from build123d import *

# Parameters (mm, degrees)
BOSS_EXTRUDE1_DEPTH = 10
SKETCH2_R           = 2.5
CUT_EXTRUDE1_DEPTH  = 10
SKETCH4_R           = 1.7
CUT_EXTRUDE4_DEPTH  = 20
CHAMFER1_SIZE       = 2.5
CHAMFER2_SIZE       = 1


with BuildPart() as part:
    # Sketch1 → Boss-Extrude1 (new body)
    with BuildSketch(Plane(origin=(0, 0, 0), x_dir=(1, 0, 0), z_dir=(0, 1, 0))):
        Polygon((-5, 5), (-5, 3), (-30, 3), (-30, -3), (-5, -3), (-5, -5), (5, -5), (5, 5), align=None)
    extrude(amount=BOSS_EXTRUDE1_DEPTH)

    # Sketch2 → Cut-Extrude1 (cut)
    with BuildSketch(Plane(origin=(0, 10, 0), x_dir=(1, 0, 0), z_dir=(0, 1, 0))):
        with Locations(Location((0, 0, 0), (0, 0, 270))):
            Circle(SKETCH2_R)
    extrude(amount=-CUT_EXTRUDE1_DEPTH, mode=Mode.SUBTRACT)

    # Sketch4 → Cut-Extrude4 (cut)
    with BuildSketch(Plane.ZY.offset(30)):
        with Locations((0, 5)):
            Circle(SKETCH4_R)
    extrude(amount=-CUT_EXTRUDE4_DEPTH, mode=Mode.SUBTRACT)

    # Chamfer1
    # the kernel refuses this chamfer: 2.5 mm, written as the material it takes off along each edge
    with BuildSketch(Plane(origin=(5, -6.42920747, -5), x_dir=(-0.9996219169112968, 0, -0.027495876610586317), z_dir=(0, 1, 0)), Plane(origin=(5, -6.42920747, 5), x_dir=(0.027495876610586317, 0, -0.9996219169112968), z_dir=(0, 1, 0))) as chamfer1_piece_1:
        Polygon((CHAMFER1_SIZE * 0.999621916911, CHAMFER1_SIZE * 0.0274958766106), (-CHAMFER1_SIZE * 0.0274958766106, CHAMFER1_SIZE * 0.999621916911), (0, 0), align=None)
    extrude(amount=22.85841494, mode=Mode.SUBTRACT)
    with BuildSketch(Plane(origin=(-5, -6.42920747, 5), x_dir=(0.9996219169112968, 0, 0.027495876610586317), z_dir=(0, 1, 0))) as chamfer1_piece_2_section:
        Polygon((CHAMFER1_SIZE * 0.999621916911, CHAMFER1_SIZE * 0.0274958766106), (-CHAMFER1_SIZE * 0.0274958766106, CHAMFER1_SIZE * 0.999621916911), (0, 0), align=None)
    chamfer1_piece_2 = extrude(amount=22.85841494, mode=Mode.PRIVATE)
    chamfer1_piece_2 = split(chamfer1_piece_2, bisect_by=Plane(origin=(-4.135703969, 5, 3), z_dir=(0, 0, 1)), keep=Keep.TOP, mode=Mode.PRIVATE)
    add(chamfer1_piece_2, mode=Mode.SUBTRACT)
    with BuildSketch(Plane(origin=(-5, -6.42920747, -5), x_dir=(-0.027495876610588735, 0, 0.9996219169112968), z_dir=(0, 1, 0))) as chamfer1_piece_3_section:
        Polygon((CHAMFER1_SIZE * 0.999621916911, CHAMFER1_SIZE * 0.0274958766106), (-CHAMFER1_SIZE * 0.0274958766106, CHAMFER1_SIZE * 0.999621916911), (0, 0), align=None)
    chamfer1_piece_3 = extrude(amount=22.85841494, mode=Mode.PRIVATE)
    chamfer1_piece_3 = split(chamfer1_piece_3, bisect_by=Plane(origin=(-4.135703969, 5, -3), z_dir=(0, 0, -1)), keep=Keep.TOP, mode=Mode.PRIVATE)
    add(chamfer1_piece_3, mode=Mode.SUBTRACT)

    # Chamfer2
    chamfer2_edges = [part.edges().sort_by_distance(p)[0] for p in [
        (-17.25, 10, -3),
        (-17.25, 10, 3),
        (-17.25, 0, 3),
        (-17.25, 0, -3),
    ]]
    chamfer(chamfer2_edges, length=CHAMFER2_SIZE)


solid = part.part
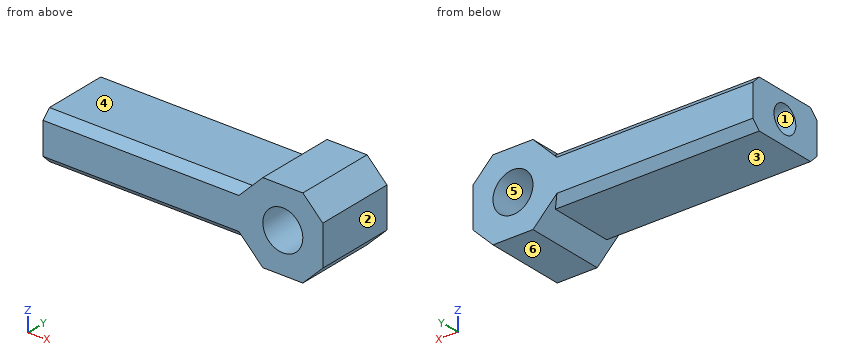
Verification items for the finished model (mm, model axes). Face numbers are marked on the shaded views. A direction names the side the tool comes from. Coordinates: 2 decimals unless noted, no trailing zeros. Order: outer loops, then holes, each group sorted by start corner. A loop starts at its lowest first (then second) coordinate and runs counter-clockwise, first axis right, second up. Notation, with made-up numbers: M 61.25,82 L 83.25,82 A23 cw 83.25,95 Z; hole C 70.5,80 d3. An arc over 180 degrees is marked long. One line per item, written item: value. Start each with the question number.
Item 1: Thickness scan on probe 1 along X at (y, z) = (3.25, 0); probe 2 along Y at (x, z) = (-14.75, 0); probe 3 along Z at (x, y) = (-28, 7). Record the ranges inside material, lowest first.
Item 2: Mould release check, pull along Z, two halves, no side actions. Record for the marked faces 4, 5 and 6: pulls with the +Z half, pulls with the -Z half, needs draft (parallel to the pull), parting line crosses it, or undercut.
Item 3: Depth check by flat-ended pin: P1, Ø1.5, axis at x = -4.5, y = 1, coming from the -Z side; P2, Ø2.5, axis at y = 5, z = 0, coming from the -X side; P3, Ø4, axis at x = -18, y = 5, coming from the -Z side. Enter the tip coordinate at first touch or a pass-through.
Item 4: Sectioned sample at B-B on y = 5. Record the cut outline in (x, z).
Item 5: Sectioned sample at A-A on x = 0. Record the cut outline in (y, z).
Item 6: Access from +Z, -Z, +X, -X, +Y, -Y to the whole of each face (thin tool, end or side, straight path). Record for the marked faces 1, 2 and 3.
Item 7: Sectioned sample at C-C on z = 0. Record the cut outline in (x, y).
Item 8: Sectioned sample at D-D on x = -7.5. Record the cut outline in (y, z), then the cut area to 3 significant figures.
Calculated:
1. probe 1: -30 to -2.5, 2.5 to 5
1. probe 2: 0 to 3.3, 6.7 to 10
1. probe 3: -3 to 3
2. face 4: pulls with the +Z half
2. face 5: undercut
2. face 6: pulls with the -Z half
3. P1: z = -3.75
3. P2: x = -10
3. P3: z = -3
4. outline: M -30,-3 L -4.5,-3 L -2.5,-5 L 2.5,-5 L 5,-2.5 L 5,2.5 L 2.5,5 L -2.5,5 L -4.5,3 L -30,3 L -30,1.7 L -10,1.7 L -10,-1.7 L -30,-1.7 Z; hole C 0,0 d5
5. outline: M 0,-5 L 10,-5 L 10,-2.5 L 0,-2.5 Z; M 0,2.5 L 10,2.5 L 10,5 L 0,5 Z
6. face 1: -X
6. face 2: +Z, -Z, +X, +Y, -Y
6. face 3: -Z, -X, +Y, -Y
7. outline: M -30,0 L -2.5,0 L -2.5,10 L -30,10 L -30,6.7 L -10,6.7 L -10,3.3 L -30,3.3 Z; M 2.5,0 L 5,0 L 5,10 L 2.5,10 Z
8. outline: M 0,-2 L 1,-3 L 9,-3 L 10,-2 L 10,2 L 9,3 L 1,3 L 0,2 Z
8. area: 58.0 mm^2
